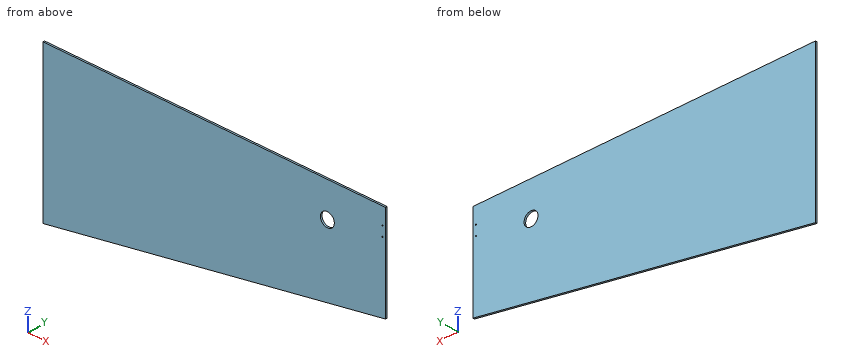
Autodesk Inventor part; units mm, degrees
ref_plane "YZ Plane" through (0, 0, 0) normal (1, 0, 0) x (0, 1, 0)
ref_plane "XZ Plane" through (0, 0, 0) normal (0, 1, 0) x (-1, 0, 0)
ref_plane "XY Plane" through (0, 0, 0) normal (0, 0, 1) x (1, 0, 0)
sketch "Sketch1" plane through (0, 0, 0) normal (0, 1, 0) x (-1, 0, 0)
  line L0 (0, 0) -> (-590, 0)
  line L1 (-590, 0) -> (-590, -165.9671)
  line L2 (-590, -165.9671) -> (0, -165.9671)
  line L3 (0, -165.9671) -> (0, 0)
  line L4 (0, -165.9671) -> (0, -270)
  line L5 (0, -270) -> (-590, -165.9671)
  dimension "d0" = 590
  dimension "d28" = 270
  dimension "d29" = 10
extrude "Extrusion1" add sketch "Sketch1" along normal blind 3
sketch "Sketch3" plane through (0, 3, 0) normal (0, 1, 0) x (1, 0, 0)
  circle A0 centre (585, 29) radius 1
  circle A1 centre (585, 46) radius 1
  line L0 (590, 0) -> (590, 165.9671)
  line L1 (0, 0) -> (590, 0)
  dimension "d15" = 2
  dimension "d16" = 5
  dimension "d17" = 5
  dimension "d18" = 2
  dimension "d19" = 29
  dimension "d20" = 17
extrude "Extrusion3" cut sketch "Sketch3" along normal through all both and the other way through all
sketch "Sketch4" plane through (0, 3, 0) normal (0, 1, 0) x (1, 0, 0)
  circle A0 centre (490, 60) radius 12
  line L0 (0, 0) -> (590, 0)
  line L1 (590, 0) -> (590, 165.9671)
  dimension "d23" = 24
  dimension "d24" = 60
  dimension "d25" = 100
extrude "Extrusion4" cut sketch "Sketch4" against normal through all
equation "\"d17\" = d16"
equation "\"d18\" = d15"
properties part number "pinball-case-left-wall-outer"
Here's how the part is built. I have some questions about the finished solid (model axes, mm). Coordinates: 2 decimals unless noted, no trailing zeros. Order: outer loops, then holes, each group sorted by start corner. A loop starts at its lowest first (then second) coordinate and runs counter-clockwise, first axis right, second up. Notation, with made-up numbers: M 87.5,66 L 123.5,66 A22 cw 123.5,74 Z; hole C 14,74.25 d1. An arc over 180 degrees is marked long. Answer as CSV lines item,"result".
Item 1: For pin 1 (12 mm diameter, centred on x = 480, z = -103, fed in from -Y), with a flat end and sliding along its axis, tell me the tip position at first contact or that it passes through.
Results found:
pin 1,"y = 0"
Item 2: Imagine slicing it at A-A on z = -60. Write out the boundary of the cut face in (x, y).
Results found:
outline,"M 0,0 L 478,0 L 478,3 L 0,3 Z; M 502,0 L 590,0 L 590,3 L 502,3 Z"
Item 3: Imagine slicing it at C-C on x = 490. Write out the boundary of the cut face in (y, z), plus the area to 3 significant figures.
Results found:
outline,"M 0,-183.6 L 3,-183.6 L 3,-72 L 0,-72 Z; M 0,-48 L 3,-48 L 3,0 L 0,0 Z"
area,"479 mm2"
Item 4: Imagine slicing it at D-D on x = 303. Write out the boundary of the cut face in (y, z).
Results found:
outline,"M 0,-216.57 L 3,-216.57 L 3,0 L 0,0 Z"
Item 5: If I drill on line 1 (X direction, y = 1.3, z = -46); line 2 (X direction, y = 1.35, z = -60); line 3 (Z direction, x = 585, y = 0.8), over which ranges is the centre line in solid material (lowest first)?
Results found:
line 1,"0 to 584, 586 to 590"
line 2,"0 to 478, 502 to 590"
line 3,"-166.85 to -47, -45 to -30, -28 to 0"
Item 6: Imagine slicing it at B-B on y = 1.9. Write out the boundary of the cut face in (x, z).
Results found:
outline,"M 0,-270 L 590,-165.97 L 590,0 L 0,0 Z; hole C 490,-60 d24; hole C 585,-46 d2; hole C 585,-29 d2"
